from build123d import *

# Parameters (mm, degrees)
SKETCH_1_R      = 1.670194834
EXTRUDE_1_DEPTH = 3


with BuildPart() as part:
    # 草图1 → 凸台-拉伸1 (new body)
    with BuildSketch(Plane(origin=(0, 0, 0), x_dir=(1, 0, 0), z_dir=(0, 1, 0))):
        Polygon((-14.3760191, 4.830077554), (-14.3760191, -2.722447763), (-24.3760191, -2.722447763), (-24.3760191, -12.722447763), (-9.3760191, -12.722447763), (-9.3760191, -7.722447763), (1.8739809, -7.722447763), (1.8739809, -12.722447763), (14.3739809, -12.722447763), (14.3739809, -7.722447763), (25.6239809, -7.722447763), (25.6239809, -12.722447763), (40.6239809, -12.722447763), (40.6239809, 2.077552237), (25.6239809, 2.077552237), (25.6239809, 14.327552237), (-15.0260191, 54.977552237), (-39.774756442, 30.228814896), align=None)
        with Locations(Location((-20.806617036, 42.903703948, 0), (0, 0, 270))):
            Circle(SKETCH_1_R, mode=Mode.SUBTRACT)
        with Locations(Location((-27.700908153, 36.009412832, 0), (0, 0, 90))):
            Circle(SKETCH_1_R, mode=Mode.SUBTRACT)
        with Locations(Location((6.664481413, 1.644023266, 0), (0, 0, 270))):
            Circle(SKETCH_1_R, mode=Mode.SUBTRACT)
        with Locations(Location((13.558772529, 8.538314383, 0), (0, 0, 90))):
            Circle(SKETCH_1_R, mode=Mode.SUBTRACT)
        Polygon((0, 0), (15.202795796, 15.202795796), (-14.142135624, 44.547727215), (-29.344931419, 29.344931419), align=None, mode=Mode.SUBTRACT)
    extrude(amount=EXTRUDE_1_DEPTH)


solid = part.part
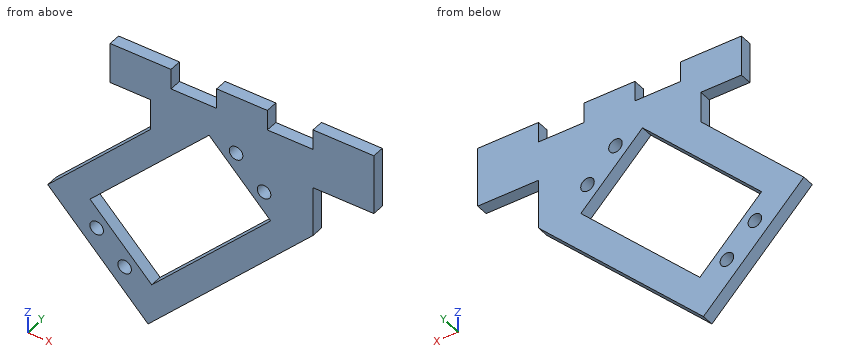
Work out the finished part from the listing and answer in its coordinate system (mm). Give positions to 0.01 mm unless a question says otherwise; leave off trailing zeros. Loops run counter-clockwise (first coordinate to the right, second up) from the corner with the lowest first, then second, coordinate; pieces in that order, holes last. Notation, with made-up numbers: M 83.5,58.25 L 89.5,58.25 A7 cw 89.5,64.25 Z; hole C 18,62 d11. An arc over 180 degrees is marked long. Use CSV: the item, a comma, the result in double quotes.
1) Find section B-B on y = 1.35. Write down the section's boundary in (x, z).
Answer:
outline,"M -39.77,-30.23 L -15.03,-54.98 L 25.62,-14.33 L 25.62,-2.08 L 40.62,-2.08 L 40.62,12.72 L 25.62,12.72 L 25.62,7.72 L 14.37,7.72 L 14.37,12.72 L 1.87,12.72 L 1.87,7.72 L -9.38,7.72 L -9.38,12.72 L -24.38,12.72 L -24.38,2.72 L -14.38,2.72 L -14.38,-4.83 Z; hole C -27.7,-36.01 d3.34; hole M -29.34,-29.34 L -14.14,-44.55 L 15.2,-15.2 L 0,0 Z; hole C -20.81,-42.9 d3.34; hole C 6.66,-1.64 d3.34; hole C 13.56,-8.54 d3.34"
2) Given P1, Ø1.5, axis at x = -18.5, y = 1.5, coming from the -Z side; P2, Ø0.9, axis at x = -3.5, y = 1, coming from the +Z side; P3, Ø1.5, axis at y = 1, z = 11.5, coming from the -X side, each flat-ended and moving along its own axis, determine where each tip first touches the part or whether it passes through.
Answer:
P1,"z = -52.25"
P2,"z = 7.72"
P3,"x = -24.38"
3) Find section A-A on z = -28.5. Write down the section's boundary in (x, y).
Answer:
outline,"M -38.05,0 L -28.5,0 L -28.5,3 L -38.05,3 Z; M 1.91,0 L 11.45,0 L 11.45,3 L 1.91,3 Z"
4) Consider L1, parallel to X at y = 2.75, z = 8; L2, parallel to Z at x = -16.5, y = 1.65; L3, parallel to X at y = 0.2, z = -36. Determine where each line is inside the solid, lowest interval first.
Answer:
L1,"-24.38 to -9.38, 1.87 to 14.37, 25.62 to 40.62"
L2,"-53.5 to -42.19, -16.5 to -6.95, 2.72 to 12.72"
L3,"-34 to -29.37, -26.03 to -22.69, -5.59 to 3.95"
5) Find section C-C on x = 3.5. Write down the section's boundary in (y, z), plus the area to 3 significant figures.
Answer:
outline,"M 0,-36.45 L 3,-36.45 L 3,-26.91 L 0,-26.91 Z; M 0,-3.5 L 3,-3.5 L 3,12.72 L 0,12.72 Z"
area,"77.3 mm^2"
6) Find section D-D on z = -43.5. Write down the section's boundary in (x, y).
Answer:
outline,"M -26.5,0 L -22.37,0 L -22.37,3 L -26.5,3 Z; M -19.25,0 L -15.19,0 L -15.19,3 L -19.25,3 Z; M -13.09,0 L -3.55,0 L -3.55,3 L -13.09,3 Z"
